The listing builds one solid part. Answer for the finished solid, in the listing's coordinates (mm). Face numbers are marked on the shaded views. Give positions to 0.01 mm unless a question says otherwise; leave off trailing zeros. Order: outer loops, then holes, each group sorted by start corner. A loop starts at its lowest first (then second) coordinate and runs counter-clockwise, first axis right, second up. Notation, with made-up numbers: (-10, 4.5) - (36, 4.5) arc R22 cw to (36, 17.5) - close; hole circle Ø3 at (68, -9). An arc over 180 degrees is marked (long way). Answer in a Markdown table with one row per item.
from build123d import *

# Parameters (mm, degrees)
SKETCH_1_W      = 57
SKETCH_1_H      = 12.35
SKETCH_2_R      = 3.5
EXTRUDE_1_DEPTH = 2
SKETCH_5_R      = 0.75
EXTRUDE_3_DEPTH = 4
SKETCH_6_R      = 6.7
EXTRUDE_4_DEPTH = 4
EXTRUDE_5_DEPTH = 9


with BuildPart() as part:
    # Эскиз1 → Повернуть1 (revolve)
    with BuildSketch(Plane(origin=(0, 0, 0), x_dir=(1, 0, 0), z_dir=(0, 1, 0)), mode=Mode.PRIVATE) as revolve_1_sk:
        with Locations((0, 6.175)):
            Rectangle(SKETCH_1_W, SKETCH_1_H)
    revolve(revolve_1_sk.sketch.rotate(Axis((-28.5, 0, 0), (1, 0, 0)), 180), axis=Axis((-28.5, 0, 0), (1, 0, 0)))

    # Эскиз2 → Бобышка-Вытянуть1 (add)
    with BuildSketch(Plane(origin=(28.5, 0, 0), x_dir=(0, 0, -1), z_dir=(1, 0, 0))):
        with Locations(Location((0, 0, 0), (0, 0, 180))):
            Circle(SKETCH_2_R)
    extrude(amount=EXTRUDE_1_DEPTH)

    # Эскиз5 → Бобышка-Вытянуть3 (add)
    with BuildSketch(Plane.ZY.offset(28.5)):
        with Locations(Location((0, 0, 0), (0, 0, 180))):
            Circle(SKETCH_5_R)
    extrude(amount=EXTRUDE_3_DEPTH)

    # Эскиз6 → Бобышка-Вытянуть4 (add)
    with BuildSketch(Plane.ZY.offset(32.5)):
        Circle(SKETCH_6_R)
    extrude(amount=EXTRUDE_4_DEPTH)

    # Эскиз3 → Бобышка-Вытянуть5 (add)
    with BuildSketch(Plane(origin=(30.5, 0, 0), x_dir=(0, 0, -1), z_dir=(1, 0, 0))):
        with BuildLine():
            Line((1.183215957, 1.55), (-1.183215957, 1.55))
            ThreePointArc((-1.183215957, 1.55), (-0.864647004, -1.747823091), (1.95, 0))
            ThreePointArc((1.95, 0), (1.747823091, 0.864647004), (1.183215957, 1.55))
        make_face()
    extrude(amount=EXTRUDE_5_DEPTH)


solid = part.part
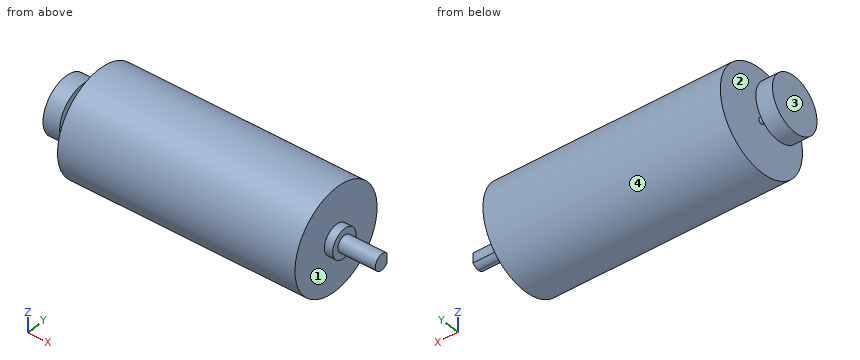
Item 1: Find section D-D on y = -8.75. Write down the section's boundary in (x, z).
Answer block:
| item | result |
|---|---|
| outline | (-28.5, -8.72) - (28.5, -8.72) - (28.5, 8.72) - (-28.5, 8.72) - close |
Item 2: Consider line 1 (Y direction, x = -18, z = 0.5); line 2 (X direction, y = -3.75, z = 1); line 3 (X direction, y = -6.5, z = 2.5). Determine where each line is inside the solid, lowest interval first.
Answer block:
| item | result |
|---|---|
| line 1 | -12.34 to 12.34 |
| line 2 | -36.5 to -32.5, -28.5 to 28.5 |
| line 3 | -28.5 to 28.5 |
Item 3: Find section C-C on x = 7. Write down the section's boundary in (y, z).
Answer block:
| item | result |
|---|---|
| outline | circle Ø24.7 at (0, 0) |
Item 4: Each of these flat-tipped pins is pushed along its axis until it touches: P1, Ø10, axis at x = 12.5, y = -9, coming from the -Z side; P2, Ø3, axis at x = -1.5, z = -6, coming from the -Y side; P3, Ø1.5, axis at x = 13, z = 8.5, coming from the -Y side. Where does it stop, or does it pass through?
Answer block:
| item | result |
|---|---|
| P1 | z = -11.68 |
| P2 | y = -11.5 |
| P3 | y = -9.62 |
Item 5: Determine the mould class of the marked faces 1, 2, 3 and 4 for opening direction X: pulls with the +X half, pulls with the -X half, needs draft (parallel to the pull), parting line crosses it, or undercut.
Answer block:
| item | result |
|---|---|
| face 1 | pulls with the +X half |
| face 2 | undercut |
| face 3 | pulls with the -X half |
| face 4 | needs draft |
Item 6: Find section A-A on z = 0. Write down the section's boundary in (x, y), then the cut area to 3 significant figures.
Answer block:
| item | result |
|---|---|
| outline | (-36.5, -6.7) - (-32.5, -6.7) - (-32.5, -0.75) - (-28.5, -0.75) - (-28.5, -12.35) - (28.5, -12.35) - (28.5, -3.5) - (30.5, -3.5) - (30.5, -1.95) - (39.5, -1.95) - (39.5, 1.55) - (30.5, 1.55) - (30.5, 3.5) - (28.5, 3.5) - (28.5, 12.35) - (-28.5, 12.35) - (-28.5, 0.75) - (-32.5, 0.75) - (-32.5, 6.7) - (-36.5, 6.7) - close |
| area | 1,510 mm² |
Item 7: Find section B-B on y = 5.75. Write down the section's boundary in (x, z).
Answer block:
| item | result |
|---|---|
| outline | (-36.5, -3.44) - (-32.5, -3.44) - (-32.5, 3.44) - (-36.5, 3.44) - close; (-28.5, -10.93) - (28.5, -10.93) - (28.5, 10.93) - (-28.5, 10.93) - close |
